Can you work these out from the model? Positions are in its coordinate system, mm. Face numbers are marked on the shaded views. A direction names the side the tool comes from. Give positions to 0.01 mm unless a question says otherwise; leave off trailing zeros. Order: outer loops, then holes, each group sorted by start corner. A loop starts at its lowest first (then second) coordinate and runs counter-clockwise, first axis right, second up. Notation, with made-up numbers: (-31, 44) -> (3, 44) arc R11 cw to (3, 57) -> close; hole circle Ø5 at (-25.75, 73). An arc over 180 degrees is marked (long way). Answer as a JSON object with one key per item and string values.
```python
from build123d import *

# Parameters (mm, degrees)
SKETCH_W     = 15
SKETCH_H     = 6
PAD_DEPTH    = 8
SKETCH001_W  = 15
SKETCH001_H  = 4.7
PAD001_DEPTH = 6
SKETCH003_W  = 1.275
SKETCH003_H  = 4.7
POCKET_DEPTH = 5.5
SKETCH004_W  = 1
SKETCH004_H  = 1
PAD002_DEPTH = 3


with BuildPart() as part:
    # Sketch → Pad (new body)
    with BuildSketch(Plane.XY):
        Rectangle(SKETCH_W, SKETCH_H)
    extrude(amount=PAD_DEPTH)

    # Sketch001 (on Face6 of Pad) → Pad001 (join)
    with BuildSketch(Plane.XY.offset(8)):
        Rectangle(SKETCH001_W, SKETCH001_H)
    extrude(amount=PAD001_DEPTH)

    # Sketch003 (on Face12 of Pad001) → Pocket (cut)
    with BuildSketch(Plane.XY.offset(14)):
        with Locations((1.7875, 0)):
            Rectangle(SKETCH003_W, SKETCH003_H)
        with Locations((5.3625, 0)):
            Rectangle(SKETCH003_W, SKETCH003_H)
        with Locations((-1.7875, 0)):
            Rectangle(SKETCH003_W, SKETCH003_H)
        with Locations((-5.3625, 0)):
            Rectangle(SKETCH003_W, SKETCH003_H)
    extrude(amount=-POCKET_DEPTH, mode=Mode.SUBTRACT)

    # Sketch004 (on Face4 of Pocket) → Pad002 (join)
    with BuildSketch(Plane(origin=(0, 0, 0), x_dir=(1, 0, 0), z_dir=(0, 0, -1))):
        with Locations((-1.82, 0)):
            Rectangle(SKETCH004_W, SKETCH004_H)
        with Locations((-5.46, 0)):
            Rectangle(SKETCH004_W, SKETCH004_H)
        with Locations((1.82, 0)):
            Rectangle(SKETCH004_W, SKETCH004_H)
        with Locations((5.46, 0)):
            Rectangle(SKETCH004_W, SKETCH004_H)
    extrude(amount=PAD002_DEPTH)


solid = part.part
```
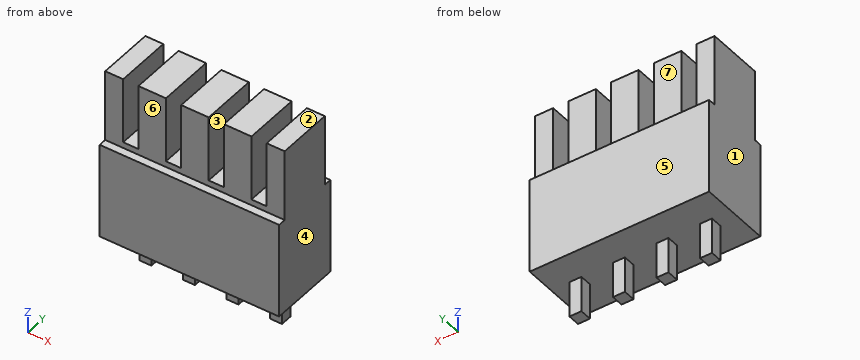
1. For the marked faces 5, 6 and 7, which set-ups out of +Z, -Z, +X, -X, +Y, -Y let a thin tool reach every point of the face, with its end or its side?
Worked answers:
{"face 5": "+Z, -Z, +X, -X, +Y", "face 6": "+Z, +X, -X, -Y", "face 7": "+Z, +X, -X, +Y"}
2. If we section it at D-D on z = 9.5: Please give me the cut outline in (x, y) (3 decimals), then the cut area to 3 significant figures.
Worked answers:
{"outline": "(-7.5, -2.35) -> (-6, -2.35) -> (-6, 2.35) -> (-7.5, 2.35) -> close; (-4.725, -2.35) -> (-2.425, -2.35) -> (-2.425, 2.35) -> (-4.725, 2.35) -> close; (-1.15, -2.35) -> (1.15, -2.35) -> (1.15, 2.35) -> (-1.15, 2.35) -> close; (2.425, -2.35) -> (4.725, -2.35) -> (4.725, 2.35) -> (2.425, 2.35) -> close; (6, -2.35) -> (7.5, -2.35) -> (7.5, 2.35) -> (6, 2.35) -> close", "area": "46.5 mm²"}
3. If we mould it in two halves opening along X, with no side actions, what happens to the marked faces 1, 2, 3 and 4? For each: +X half, -X half, draft (parallel to the pull), parting line (faces both ways), or undercut.
Worked answers:
{"face 1": "-X half", "face 2": "draft", "face 3": "undercut", "face 4": "+X half"}
4. Will these pins go through, and if not, where does the flat tip stop? pin 1 Ø0.5 at (x, z) = (5.5, -2) entering from +Y; pin 2 Ø0.5 at (y, z) = (0, -1) entering from -X; pin 3 Ø1.8 at (x, z) = (2, 12) entering from +Y.
Worked answers:
{"pin 1": "y = 0.5", "pin 2": "x = -5.96", "pin 3": "y = 2.35"}
5. If we section it at A-A on z = -0.5: Please give me the cut outline in (x, y), then the cut area to 3 significant figures.
Worked answers:
{"outline": "(-5.96, -0.5) -> (-4.96, -0.5) -> (-4.96, 0.5) -> (-5.96, 0.5) -> close; (-2.32, -0.5) -> (-1.32, -0.5) -> (-1.32, 0.5) -> (-2.32, 0.5) -> close; (1.32, -0.5) -> (2.32, -0.5) -> (2.32, 0.5) -> (1.32, 0.5) -> close; (4.96, -0.5) -> (5.96, -0.5) -> (5.96, 0.5) -> (4.96, 0.5) -> close", "area": "4.00 mm²"}
6. If we section it at B-B on x = -5.75: Please give me the cut outline in (y, z), then the cut area to 4 significant figures.
Worked answers:
{"outline": "(-3, 0) -> (-0.5, 0) -> (-0.5, -3) -> (0.5, -3) -> (0.5, 0) -> (3, 0) -> (3, 8) -> (2.35, 8) -> (2.35, 8.5) -> (-2.35, 8.5) -> (-2.35, 8) -> (-3, 8) -> close", "area": "53.35 mm²"}
7. If we section it at C-C on y = 2.1: Please give me the cut outline in (x, z) (3 decimals).
Worked answers:
{"outline": "(-7.5, 0) -> (7.5, 0) -> (7.5, 14) -> (6, 14) -> (6, 8.5) -> (4.725, 8.5) -> (4.725, 14) -> (2.425, 14) -> (2.425, 8.5) -> (1.15, 8.5) -> (1.15, 14) -> (-1.15, 14) -> (-1.15, 8.5) -> (-2.425, 8.5) -> (-2.425, 14) -> (-4.725, 14) -> (-4.725, 8.5) -> (-6, 8.5) -> (-6, 14) -> (-7.5, 14) -> close"}
8. Please list where these lines run through material, in increasing order: L1, parallel to X at y = 0.2, z = -0.5; L2, parallel to X at y = -0.75, z = 13.25 (3 decimals); L3, parallel to Z at x = 2.5, y = -0.9.
Worked answers:
{"L1": "-5.96 to -4.96, -2.32 to -1.32, 1.32 to 2.32, 4.96 to 5.96", "L2": "-7.5 to -6, -4.725 to -2.425, -1.15 to 1.15, 2.425 to 4.725, 6 to 7.5", "L3": "0 to 14"}
